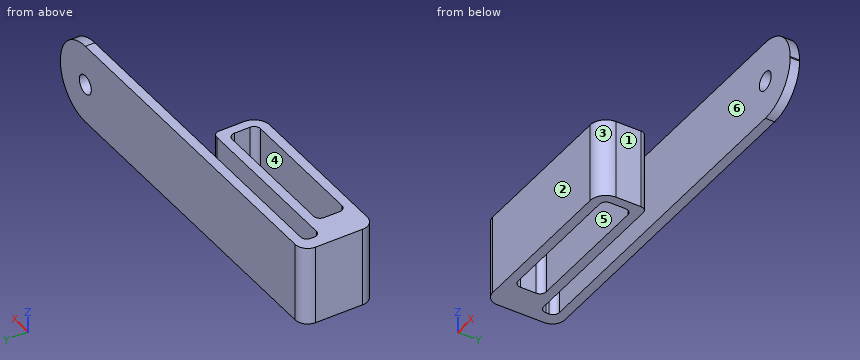
```python
from build123d import *

# Parameters (mm, degrees)
F1_DEPTH = 25.4
F3_DEPTH = 25.401
F5_DEPTH = 25.401
F6_R     = 2
F7_R     = 12.5
F8_R     = 3
F9_DEPTH = 3.001


with BuildPart() as f1:
    # F0 (on Top) → F1 (new body)
    with BuildSketch(Plane.XY):
        with BuildLine():
            Line((0, -23), (0, 0))
            Line((0, 0), (-118, 0))
            ThreePointArc((-118, 0), (-120.828427, -1.171573), (-122, -4))
            Line((-122, -4), (-122, -19))
            ThreePointArc((-122, -19), (-120.828427, -21.828427), (-118, -23))
            Line((-118, -23), (0, -23))
        make_face()
    extrude(amount=F1_DEPTH)

    # F2 (on face) → F3 (cut, through all)
    with BuildSketch(Plane.XY.offset(25.4)):
        with BuildLine():
            Line((-69, -11), (-110, -11))
            ThreePointArc((-110, -11), (-111.414214, -11.585786), (-112, -13))
            Line((-112, -13), (-112, -18))
            ThreePointArc((-112, -18), (-111.414214, -19.414214), (-110, -20))
            Line((-110, -20), (-69, -20))
            ThreePointArc((-69, -20), (-67.585786, -19.414214), (-67, -18))
            Line((-67, -18), (-67, -13))
            ThreePointArc((-67, -13), (-67.585786, -11.585786), (-69, -11))
        make_face()
    extrude(amount=-F3_DEPTH, mode=Mode.SUBTRACT)

    # F4 (on face) → F5 (cut, through all)
    with BuildSketch(Plane.XY.offset(25.4)):
        with BuildLine():
            Line((-118, -8), (-64, -8))
            Line((-64, -8), (-64, -18))
            ThreePointArc((-64, -18), (-65.464466, -21.535534), (-69, -23))
            Line((-69, -23), (0, -23))
            Line((0, -23), (0, -3))
            Line((0, -3), (-118, -3))
            Line((-118, -3), (-118, -8))
        make_face()
    extrude(amount=-F5_DEPTH, mode=Mode.SUBTRACT)

    # F6
    f6_edges = [f1.edges().sort_by_distance(p)[0] for p in [
        (-118, -3, 12.7),
        (-118, -8, 12.7),
        (-64, -8, 12.7),
    ]]
    fillet(f6_edges, radius=F6_R)

    # F7
    f7_edges = [f1.edges().sort_by_distance(p)[0] for p in [
        (0, -1.5, 25.4),
        (0, -1.5, 0),
    ]]
    fillet(f7_edges, radius=F7_R)

    # F8 (on face) → F9 (cut, through all)
    with BuildSketch(Plane.XZ.offset(3)):
        with Locations((-12.5, 12.5)):
            Circle(F8_R)
    extrude(amount=-F9_DEPTH, mode=Mode.SUBTRACT)


solid = f1.part
```
Could you check a few things on this model? Use its own coordinates, in mm. Face numbers are marked on the shaded views. A direction names the side the tool comes from. Round coordinates to 2 decimals unless told otherwise and drop trailing zeros. Write each loop counter-clockwise with the first axis right and the second up, starting at its lowest first coordinate (ties: lowest second). Pieces come first, ordered by that corner, then holes. Notation, with made-up numbers: M -21.75,58.25 L 26.25,58.25 A22 ccw 26.25,92.25 Z; hole C 22,57 d1. An arc over 180 degrees is marked long. Answer in a Markdown table with one row per item. Add a question column.
Q1. On a 3-axis mill with a long thin cutter (end or side, diameter ignored), from which of +Z, -Z, +X, -X, +Y, -Y can I reach the whole of each face in a straight line? I mean the marked faces 1 and 2. Say none if no direction works.
Q2. Will these pins go through, and if not, where does the flat tip stop? pin 1 Ø1.5 at (y, z) = (-14, 18) entering from +X; pin 2 Ø2 at (y, z) = (-6.5, 18) entering from +X; pin 3 Ø0.8 at (y, z) = (-5.5, 14) entering from +X.
Q3. If we mould it in two halves opening along X, with no side actions, what happens to the marked faces 3, 4, 5 and 6? For each: +X half, -X half, draft (parallel to the pull), parting line (faces both ways), or undercut.
Q4. If I drill on line 1 (Y direction, x = -92, z = 9.5); line 2 (X direction, y = -17, z = 21.5); line 3 (Y direction, x = -114, z = 11.25), over which ranges is the centre line in solid material (lowest first)? Write a range as from..to.
Q5. Imagine slicing it at A-A (x = -98.5). Please give me the cut outline in (y, z).
Values:
| question | item | result |
|---|---|---|
| 1 | face 1 | +Z, -Z, +X, -Y |
| 1 | face 2 | +Z, -Z, +X, -X, -Y |
| 2 | pin 1 | x = -64 |
| 2 | pin 2 | x = -117.32 |
| 2 | pin 3 | x = -118 |
| 3 | face 3 | +X half |
| 3 | face 4 | undercut |
| 3 | face 5 | undercut |
| 3 | face 6 | draft |
| 4 | line 1 | -23..-20, -11..-8, -3..0 |
| 4 | line 2 | -122..-112, -67..-64 |
| 4 | line 3 | -23..-8, -3..0 |
| 5 | outline | M -23,0 L -20,0 L -20,25.4 L -23,25.4 Z; M -11,0 L -8,0 L -8,25.4 L -11,25.4 Z; M -3,0 L 0,0 L 0,25.4 L -3,25.4 Z |
